Verification items for the finished model (mm, model axes). A direction names the side the tool comes from. Coordinates: 2 decimals unless noted, no trailing zeros. Answer in a Markdown table with one row per item.
```python
from build123d import *

# Parameters (mm, degrees)
MOUNTING_HOLE_PATTERN_COUNT = 4
SKETCH9_R                   = 12.3825
SHAFT_DIA_DEPTH             = 0.254


with BuildPart() as part:
    # Sketch1 → BASE-FLANGE (revolve)
    with BuildSketch(Plane.XY, mode=Mode.PRIVATE) as base_flange_sk:
        Polygon((-30.1625, -11.1125), (23.8125, -11.1125), (23.8125, -22.225), (30.1625, -22.225), (30.1625, -6.35), (-30.1625, -6.35), align=None)
    revolve(base_flange_sk.sketch.rotate(Axis((-10.390811595, 0, 0), (1, 0, 0)), 270), axis=Axis((-10.390811595, 0, 0), (1, 0, 0)))  # turned: the seam where the file's is

    # Sketch10 → MOUNTING-HOLE (revolve, cut)
    with BuildSketch(Plane.XY, mode=Mode.PRIVATE) as mounting_hole_sk:
        Polygon((30.1625, 20.43938), (25.79624, 20.43938), (25.79624, 19.05), (23.8125, 19.05), (23.8125, 16.66875), (30.1625, 16.66875), align=None)
    mounting_hole = revolve(mounting_hole_sk.sketch.rotate(Axis((7.205320248, 16.66875, 0), (1, 0, 0)), 90), axis=Axis((7.205320248, 16.66875, 0), (1, 0, 0)), mode=Mode.SUBTRACT)  # turned: the seam where the file's is

    # MOUNTING-HOLE PATTERN: MOUNTING-HOLE ×4 about axis
    mounting_hole_pattern_axis = Axis((0, 0, 0), (1, 0, 0))
    for i in range(1, MOUNTING_HOLE_PATTERN_COUNT):
        add(mounting_hole.rotate(mounting_hole_pattern_axis, i * 360 / MOUNTING_HOLE_PATTERN_COUNT), mode=Mode.SUBTRACT)

    # Sketch9 → SHAFT DIA (cut)
    with BuildSketch(Plane(origin=(30.1625, 0, 0), x_dir=(0, 0, -1), z_dir=(1, 0, 0))):
        Circle(SKETCH9_R)
    extrude(amount=-SHAFT_DIA_DEPTH, mode=Mode.SUBTRACT)


solid = part.part
```
1. Material ranges on probe 1 along Y at (x, z) = (-7, 0); probe 2 along X at (y, z) = (-9.5, 7.5); probe 3 along Y at (x, z) = (14, 5), recorded low to high. Write a range as from..to.
Findings below:
| item | result |
|---|---|
| probe 1 | y = -11.11..-6.35, 6.35..11.11 |
| probe 2 | x = 23.81..29.91 |
| probe 3 | y = -9.92..-3.91, 3.91..9.92 |
2. Access from +Z, -Z, +X, -X, +Y, -Y to the whole of each face (thin tool, end or side, straight path). Record for faces 4 (the face through (-2.797, -9.37, 5.974)), 5 (the face through (24.79, 1.1, -18.78)), 6 (the face through (27.95, -12.93, 0.49)).
Findings below:
| item | result |
|---|---|
| face 4 | -X |
| face 5 | +X, -X |
| face 6 | +X |
3. Sectioned sample at A-A, the plane y = 0. Count the separate pieces of the cut face and the enclosed holes in it, and give its area (3 significant figures).
Findings below:
| item | result |
|---|---|
| separate pieces | 4 |
| enclosed holes | 0 |
| area | 628 mm² |
4. Go/stop test with flat-tipped pins: pin 1 (6 mm diameter, centred on y = 0, z = 16.67, fed in from -X); pin 2 (8 mm diameter, centred on x = -3.5, z = -11.5, fed in from -Y); pin 3 (10 mm diameter, centred on x = -3.5, y = -11.5, fed in from -Z). Record where each tip stops, or that it passes through.
Findings below:
| item | result |
|---|---|
| pin 1 | stops at x = 23.81 |
| pin 2 | stops at y = -8.2 |
| pin 3 | stops at z = -9.01 |
5. Release check for a two-part mould opening along Z. For faces 1 (the face through (24.79, -1.1, 18.78)), 2 (the face through (27.03, -18.74, 11.95)), 3 (the face through (30.162, 10, 10)) record: released by +Z, released by -Z, zero draft, split by the parting line, or undercut.
Findings below:
| item | result |
|---|---|
| face 1 | undercut |
| face 2 | split by the parting line |
| face 3 | zero draft |
